Work out the finished part from the listing and answer in its coordinate system (mm). Coordinates: 2 decimals unless noted, no trailing zeros. Loops run counter-clockwise (first coordinate to the right, second up) from the corner with the lowest first, then second, coordinate; pieces in that order, holes last. Notation, with made-up numbers: M 80.5,44.5 L 139.5,44.5 A22 cw 139.5,67.5 Z; hole C 68.5,53.5 d8. An arc over 180 degrees is marked long. Write each question's results on one line, items separated by ' | '.
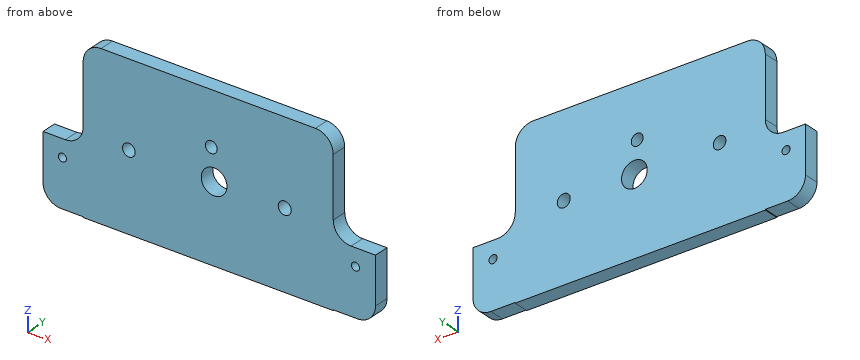
```python
from build123d import *

# Parameters (mm, degrees)
F0_R     = 1.796742
F0_R_2   = 3.661721
F0_R_3   = 1.853658
F0_R_4   = 1.683803
F0_W     = 11.430001
F0_H     = 18.327412
F0_R_5   = 1.149098
F0_W_2   = 12.02121
F0_R_6   = 1.149206
F1_DEPTH = 4.318
F2_R     = 5.08


with BuildPart() as f1:
    # F0 (on Front) → F1 (new body)
    with BuildSketch(Plane.XZ):
        Polygon((41.088879, 23.746809), (-30.053018, 23.746809), (-30.053018, -3.448707), (-30.053018, -21.776119), (-30.053018, -21.973191), (41.088879, -21.973191), (41.088879, -21.776119), (41.088879, -3.448707), align=None)
        with Locations((-17.051516, 0)):
            Circle(F0_R, mode=Mode.SUBTRACT)
        with Locations((7.193016, 0)):
            Circle(F0_R_2, mode=Mode.SUBTRACT)
        with Locations((27.29243, 0)):
            Circle(F0_R_3, mode=Mode.SUBTRACT)
        with Locations((6.401504, 8.764441)):
            Circle(F0_R_4, mode=Mode.SUBTRACT)
        with Locations((-35.768018, -12.612413)):
            Rectangle(F0_W, F0_H)
        with Locations((-35.965085, -8.375431)):
            Circle(F0_R_5, mode=Mode.SUBTRACT)
        with Locations((47.099484, -12.612413)):
            Rectangle(F0_W_2, F0_H)
        with Locations((47.395017, -8.375431)):
            Circle(F0_R_6, mode=Mode.SUBTRACT)
    extrude(amount=F1_DEPTH)

    # F2
    f2_edges = [f1.edges().sort_by_distance(p)[0] for p in [
        (-30.053018, -2.159, 23.746809),
        (41.088879, -2.159, 23.746809),
        (-30.053018, -2.159, -3.448707),
        (41.088879, -2.159, -3.448707),
        (53.110089, -2.159, -21.776119),
        (-41.483019, -2.159, -21.776119),
    ]]
    fillet(f2_edges, radius=F2_R)


solid = f1.part
```
1) Find section C-C, the plane z = 17.5. Give the vertices of the cut face in (x, y), and give its area (3 significant figures).
Check result:
outline: M -30.05,-4.32 L 41.09,-4.32 L 41.09,0 L -30.05,0 Z | area: 307 mm^2
2) Find section A-A, the plane z = 0. Give the vertices of the cut face in (x, y), and give its area (3 significant figures).
Check result:
outline: M -30.32,-4.32 L -18.85,-4.32 L -18.85,0 L -30.32,0 Z; M -15.25,-4.32 L 3.53,-4.32 L 3.53,0 L -15.25,0 Z; M 10.85,-4.32 L 25.44,-4.32 L 25.44,0 L 10.85,0 Z; M 29.15,-4.32 L 41.36,-4.32 L 41.36,0 L 29.15,0 Z | area: 246 mm^2
3) Find section B-B, the plane y = -3.6. Give the vertices of the cut face in (x, z), and give its area (3 significant figures).
Check result:
outline: M -41.48,-16.7 A5.08 ccw -36.4,-21.78 L -30.05,-21.78 L -30.05,-21.97 L 41.09,-21.97 L 41.09,-21.78 L 48.03,-21.78 A5.08 ccw 53.11,-16.7 L 53.11,-3.45 L 46.17,-3.45 A5.08 cw 41.09,1.63 L 41.09,18.67 A5.08 ccw 36.01,23.75 L -24.97,23.75 A5.08 ccw -30.05,18.67 L -30.05,1.63 A5.08 cw -35.13,-3.45 L -41.48,-3.45 Z; hole C -35.97,-8.38 d2.3; hole C -17.05,0 d3.59; hole C 7.19,0 d7.32; hole C 6.4,8.76 d3.37; hole C 27.29,0 d3.71; hole C 47.4,-8.38 d2.3 | area: 3,590 mm^2
4) Straight lines are drawn through the part: probe 1 along X at (y, z) = (-1.3, 0.5); probe 2 along X at (y, z) = (-2.3, -9); probe 3 along Z at (x, y) = (26, -3.1). For each, find the intervals that lie inside material, in ascending order. Write a range as [from, to].
Check result:
probe 1: [-30.18, -18.78], [-15.33, 3.57], [10.82, 25.51], [29.08, 41.22] | probe 2: [-41.48, -36.93], [-35, 46.43], [48.36, 53.11] | probe 3: [-21.97, -1.33], [1.33, 23.75]
5) Given pin 1 Ø3 at (x, z) = (-17.05, 0) entering from -Y; pin 2 Ø1.3 at (y, z) = (-2.5, 10.5) entering from +X, each flat-ended and moving along its own axis, determine where each tip first touches the part or whether it passes through.
Check result:
pin 1: through | pin 2: x = 41.09
